from build123d import *

# Parameters (mm, degrees)
F1_DEPTH = 6.35
F3_D     = 5.1054
F5_DEPTH = 165.1


with BuildPart() as f1:
    # F0 (on Right) → F1 (new body)
    with BuildSketch(Plane.YZ):
        with BuildLine():
            Line((25.4, 292.1), (0, 292.1))
            ThreePointArc((0, 292.1), (-206.5458907846, 206.5458907846), (-292.1, 0))
            Line((-292.1, 0), (-292.1, -25.4))
            Line((-292.1, -25.4), (-216.3804769516, -25.4))
            Line((-216.3804769516, -25.4), (-215.9, 0))
            ThreePointArc((-215.9, 0), (-152.6643540582, 152.6643540582), (0, 215.9))
            Line((0, 215.9), (25.4, 215.9))
            Line((25.4, 215.9), (25.4, 292.1))
        make_face()
    extrude(amount=F1_DEPTH)

    # F3 (through all)
    with Locations(Plane(origin=(0, 0, 0), x_dir=(0, 1, 0), z_dir=(-1, 0, 0))):
        with Locations((-170.6248663003, -170.6248663003), (-234.6654012579, -97.2015918207), (-279.4, 0), (0, -279.4), (0, -228.6), (-266.7, 0), (-188.5853785425, -188.5853785425), (-222.932131195, -92.3415122297), (-211.1988611321, -87.4814326387), (-106.9217510028, -258.1319413837), (-254, 0), (0, -266.7), (-246.3986713208, -102.0616714118), (-197.5656346635, -197.5656346635), (-228.6, 0), (-258.1319413837, -106.9217510028), (-102.0616714118, -246.3986713208), (-97.2015918207, -234.6654012579), (-161.6446101792, -161.6446101792), (-241.3, 0), (-179.6051224214, -179.6051224214), (-92.3415122297, -222.932131195), (0, 0), (0, -254), (-87.4814326387, -211.1988611321), (0, -241.3)):
            Hole(F3_D / 2)

    # F4 (on face) → F5 (join)
    with BuildSketch(Plane.YZ.offset(6.35)):
        with BuildLine():
            Line((-292.1, -25.4), (-292.1, 0))
            ThreePointArc((-292.1, 0), (-206.5458907846, 206.5458907846), (0, 292.1))
            Line((0, 292.1), (25.4, 292.1))
            Line((25.4, 292.1), (25.4, 298.45))
            Line((25.4, 298.45), (0, 298.45))
            ThreePointArc((0, 298.45), (-211.0360188451, 211.0360188451), (-298.45, 0))
            Line((-298.45, 0), (-298.45, -25.4))
            Line((-298.45, -25.4), (-292.1, -25.4))
        make_face()
    extrude(amount=-F5_DEPTH)

    # F6: F1 across face


with BuildPart() as f1_1:
    add(f1.part)
    add(f1.part.mirror(Plane(origin=(-158.75, -183.3754264806, 183.3754264806), x_dir=(0, 1, 0), z_dir=(-1, 0, 0))))


solid = f1_1.part
Model file for the job. Use its own axes, mm. A direction names the side the tool comes from. Coordinates: 2 decimals unless noted, no trailing zeros. Order: outer loops, then holes, each group sorted by start corner. A loop starts at its lowest first (then second) coordinate and runs counter-clockwise, first axis right, second up. Notation, with made-up numbers: (30.25, 65) -> (49.25, 65) arc R11 ccw to (49.25, 73) -> close; hole circle Ø1 at (-21.75, -7.5). An arc over 180 degrees is marked (long way). Return JSON: item names as keys, results as strings. Group by question number.
Item 1: Flat gauge pins, fed straight in: P1, Ø6, axis at x = -268.5, y = -240.5, coming from the +Z side; P2, Ø3, axis at x = -161, z = 147, coming from the -Y side; P3, Ø5, axis at x = -244.5, y = -206.5, coming from the +Z side. Where does each tip first touch, or does it go through?
Item 2: Saw through at A-A on x = -237. Write the cut outline in (y, z).
Item 3: Tool access for faces 1 (the cylindrical face through (-160.972, -208.804, 204.262)), 2 (the cylindrical face through (3.13, -154.33, 150.98)): list every direction of +Z, -Z, +X, -X, +Y, -Y with a clear straight run to the whole face (end or side of a thin tool).
Item 4: Wall check: line 1 along X through (y, z) = (-17, 236); line 2 along Y through (x, z) = (-289, 4.5); line 3 along Y through (x, z) = (-13.5, 7). Give the ranges that are in metal, low to high. Write a range as [from, to].
Item 5: Pull direction X, two halves, no side cores. Call faces 3 (the flat face through (-323.85, -173, 149)), 4 (the flat face through (-109, 25.4, 294)), 5 (the flat face through (-161, -292.1, -13)): pulls with the +X half, pulls with the -X half, needs draft (parallel to the pull), parting line crosses it, or undercut.
Item 6: Saw through at B-B on z = 54. Write the cut outline in (x, y).
Values found:
{
 "1": {"P1": "stops at z = 180.74", "P2": "stops at y = -260.58", "P3": "stops at z = 217.84"},
 "2": {"outline": "(-298.45, -25.4) -> (-292.1, -25.4) -> (-292.1, 0) arc R292.1 cw to (0, 292.1) -> (25.4, 292.1) -> (25.4, 298.45) -> (0, 298.45) arc R298.45 ccw to (-298.45, 0) -> close"},
 "3": {"face 1": "-Z, +Y", "face 2": "-Z, +X, -X, +Y"},
 "4": {"line 1": "x = [-323.85, -317.5], [0, 6.35]", "line 2": "y = [-298.42, -292.07]", "line 3": "y = [-298.37, -292.02]"},
 "5": {"face 3": "pulls with the -X half", "face 4": "needs draft", "face 5": "undercut"},
 "6": {"outline": "(-323.85, -293.52) -> (6.35, -293.52) -> (6.35, -209.04) -> (0, -209.04) -> (0, -287.07) -> (-317.5, -287.07) -> (-317.5, -209.04) -> (-323.85, -209.04) -> close"}
}
